Drawing for the job (mm, zero at the part's lowest x, y, z). A direction names the side the tool comes from. Coordinates: 2 decimals unless noted, no trailing zeros. Loops run counter-clockwise (first coordinate to the right, second up) from the corner with the lowest first, then second, coordinate; pieces in that order, holes last. Notation, with made-up numbers: (78.25, 83.5) -> (96.25, 83.5) arc R24 cw to (96.25, 95.5) -> close; hole circle Ø2 at (47.5, 77). An arc over 180 degrees is marked (long way). Write each question's results on one line, items separated by ' | '.
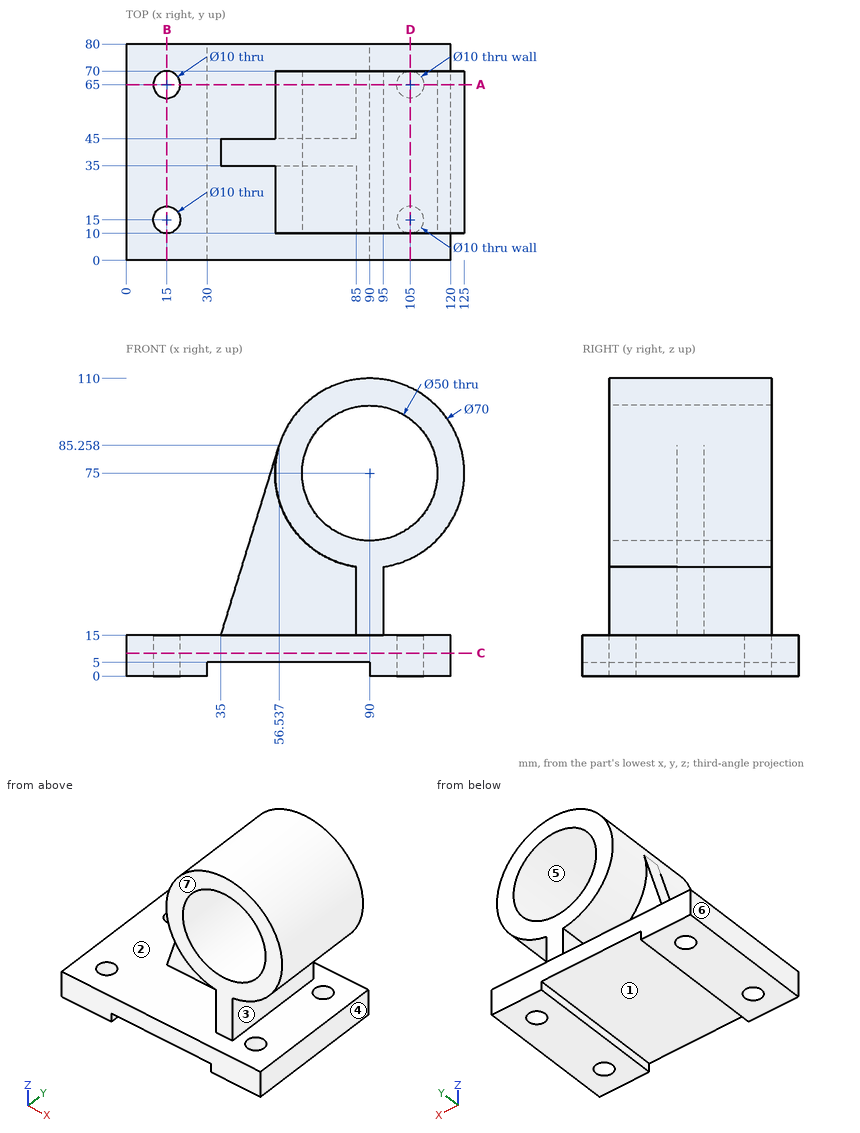
1) Slice it at A-A (y = 65). Write the cut outline in (x, z), then the cut area to 3 significant figures.
Outcome:
outline: (0, 0) -> (10, 0) -> (10, 15) -> (0, 15) -> close; (20, 0) -> (30, 0) -> (30, 5) -> (90, 5) -> (90, 0) -> (100, 0) -> (100, 15) -> (95, 15) -> (95, 40.36) arc R35 ccw (long way) to (85, 40.36) -> (85, 15) -> (20, 15) -> close; (110, 0) -> (120, 0) -> (120, 15) -> (110, 15) -> close; hole circle Ø50 at (90, 75) | area: 3,340 mm^2
2) Slice it at D-D (x = 105). Write the cut outline in (y, z), then the cut area to 3 significant figures.
Outcome:
outline: (0, 0) -> (10, 0) -> (10, 15) -> (0, 15) -> close; (10, 43.38) -> (70, 43.38) -> (70, 55) -> (10, 55) -> close; (10, 95) -> (70, 95) -> (70, 106.62) -> (10, 106.62) -> close; (20, 0) -> (60, 0) -> (60, 15) -> (20, 15) -> close; (70, 0) -> (80, 0) -> (80, 15) -> (70, 15) -> close | area: 2,290 mm^2
3) Slice it at B-B (x = 15). Write the cut outline in (y, z).
Outcome:
outline: (0, 0) -> (10, 0) -> (10, 15) -> (0, 15) -> close; (20, 0) -> (60, 0) -> (60, 15) -> (20, 15) -> close; (70, 0) -> (80, 0) -> (80, 15) -> (70, 15) -> close
4) Drill centre lines: L1, parallel to X at y = 65, z = 9; L2, parallel to Y at x = 15, z = 10.5; L3, parallel to Z at x = 113, y = 34.5. Where is each one in solid material? Low to high. Write a range as from..to.
Outcome:
L1: x = 0..10, 20..100, 110..120 | L2: y = 0..10, 20..60, 70..80 | L3: z = 0..15, 48.62..65.2, 84.8..101.38
5) Pin check, flat tips, straight feed: pin 1 (13 mm diameter, centred on x = 105, y = 15, fed in from +Z); pin 2 (5 mm diameter, centred on y = 38.5, z = 77, fed in from -X); pin 3 (16.5 mm diameter, centred on y = 47.5, z = 10.5, fed in from +X). Stop position of each tip, or through.
Outcome:
pin 1: stops at z = 108.95 | pin 2: stops at x = 53.24 | pin 3: stops at x = 120
6) Two-plate mould, pull along X, no slides. Class the marked faces 4, 5, 6 and 7: pulls with the +X half, pulls with the -X half, needs draft (parallel to the pull), parting line crosses it, or undercut.
Outcome:
face 4: pulls with the +X half | face 5: undercut | face 6: pulls with the -X half | face 7: needs draft
7) Slice it at C-C (z = 8.5). Write the cut outline in (x, y).
Outcome:
outline: (0, 0) -> (120, 0) -> (120, 80) -> (0, 80) -> close; hole circle Ø10 at (15, 15); hole circle Ø10 at (15, 65); hole circle Ø10 at (105, 15); hole circle Ø10 at (105, 65)
8) Which spindle directions (+Z, -Z, +X, -X, +Y, -Y) get a long thin tool onto all of the face, cutting with end or side? Do the marked faces 1, 2 and 3. Say none if no direction does.
Outcome:
face 1: -Z, +Y, -Y | face 2: none | face 3: +X, +Y, -Y
